Verification items for this drawing (mm, ordinates from the low corner). A direction names the side the tool comes from. Coordinates: 2 decimals unless noted, no trailing zeros. Loops run counter-clockwise (first coordinate to the right, second up) from the corner with the lowest first, then second, coordinate; pieces in that order, holes last. Notation, with made-up numbers: (-9.5, 10) - (49.5, 10) arc R21 ccw to (49.5, 32) - close; hole circle Ø5 at (40, 61). An arc over 180 degrees is marked (long way). One line per item, written item: value. Start each with the question number.
(1) Section check B-B (x = 21). Record the boundary of the cut face in (y, z).
(2) Section check C-C (z = 0.95). Count the separate pieces of the cut face and the enclosed holes in it, plus the area to 3 significant figures.
(3) Draft check along X on the marked faces 4, 5, 6 and 7. Enter one of: +X half, -X half, draft (parallel to the pull), parting line (faces both ways), or undercut.
(4) Section check A-A (y = 25.5). Record the boundary of the cut face in (x, z).
(5) Gauge pin test, flat ends, axial feed: P1, Ø0.9, axis at y = 24, z = 1, coming from the +X side; P2, Ø0.8, axis at x = 29, z = 2, coming from the +Y side. Record the tip position at first contact, or that the pin passes through.
(6) Thickness scan on probe 1 along X at (y, z) = (19.5, 0.3); probe 2 along Y at (x, z) = (20.5, 2.1). Record the ranges inside material, lowest first. Write a range as [from, to].
(7) Set-up check for the marked faces 1, 2 and 3: record each of +Z, -Z, +X, -X, +Y, -Y from which the full face is reachable in a straight line by a thin tool's end or side.
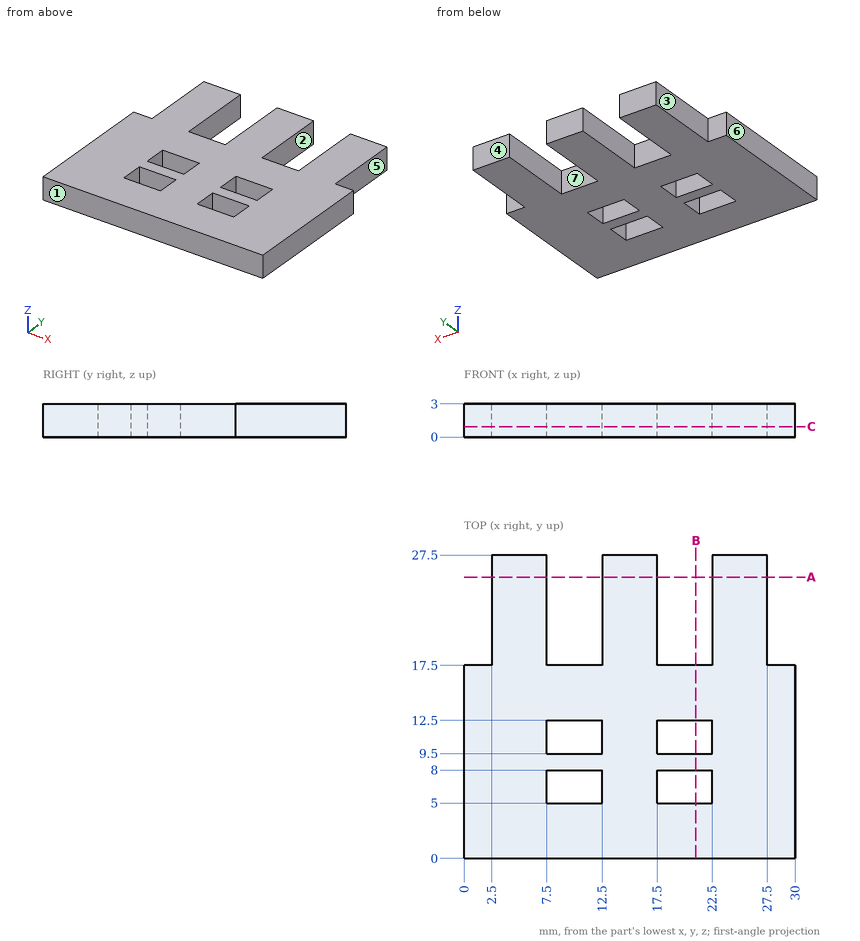
Responses:
1. outline: (0, 0) - (5, 0) - (5, 3) - (0, 3) - close; (8, 0) - (9.5, 0) - (9.5, 3) - (8, 3) - close; (12.5, 0) - (17.5, 0) - (17.5, 3) - (12.5, 3) - close
2. separate pieces: 1
2. enclosed holes: 4
2. area: 615 mm²
3. face 4: draft
3. face 5: +X half
3. face 6: -X half
3. face 7: undercut
4. outline: (2.5, 0) - (7.5, 0) - (7.5, 3) - (2.5, 3) - close; (12.5, 0) - (17.5, 0) - (17.5, 3) - (12.5, 3) - close; (22.5, 0) - (27.5, 0) - (27.5, 3) - (22.5, 3) - close
5. P1: stops at x = 27.5
5. P2: stops at y = 17.5
6. probe 1: x = [2.5, 7.5], [12.5, 17.5], [22.5, 27.5]
6. probe 2: y = [0, 5], [8, 9.5], [12.5, 17.5]
7. face 1: +Z, -Z, +X, -X, -Y
7. face 2: +Z, -Z, +Y
7. face 3: +Z, -Z, -X, +Y
